The model under review builds one solid part; all positions refer to its coordinate system, in mm. Round coordinates to 2 decimals unless told otherwise and drop trailing zeros. Loops run counter-clockwise (first coordinate to the right, second up) from the corner with the lowest first, then second, coordinate; pieces in that order, holes last. Notation, with made-up numbers: (30.25, 46) -> (68.25, 46) arc R19 cw to (68.25, 69) -> close; hole circle Ø6 at (11, 82). An arc over 180 degrees is marked (long way). Write each question's results on one line, items separated by ' | '. Start each with the question number.
Item 1: We need section C-C (x = -43). Give the boundary of the cut face in (y, z).
Item 2: We need section D-D (z = 76). Give the boundary of the cut face in (x, y), and give its area (3 significant figures).
Item 3: We need section B-B (y = 0.65). Give the number of separate pieces and of enclosed holes in the cut face, and give its area (3 significant figures).
Item 4: For L1, parallel to X at y = 0.6, z = 92.5; L2, parallel to Z at x = 75.5, y = 2.1; L3, parallel to Z at x = -77.5, y = 0.3, list the stretches that pass through material, from the lowest coordinate up. Write a range as from..to.
Item 5: We need section A-A (z = -55). Give the boundary of the cut face in (x, y), and give its area (3 significant figures).
Item 6: Clearance check with flat-ended pins moving along their axes: pin 1 Ø1 at (y, z) = (1, 59.5) entering from +X; pin 2 Ø0.8 at (x, y) = (5, 1.5) entering from -Z; pin 3 Ø0.8 at (y, z) = (1, -76.5) entering from +X. State where each tip first meets the part, or that it passes through.
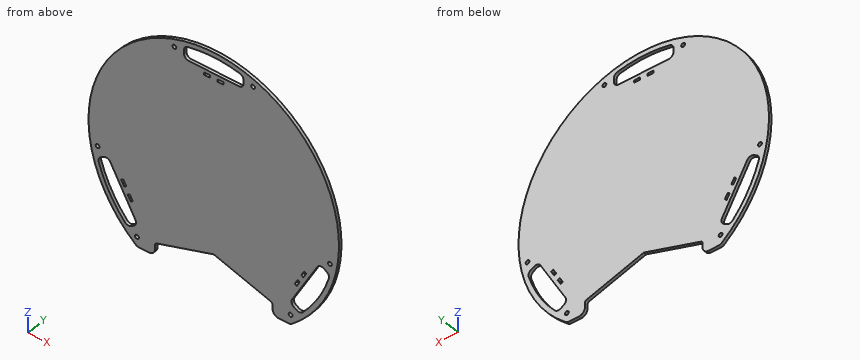
Autodesk Inventor part; units mm, degrees
ref_plane "YZ Plane" through (0, 0, 0) normal (1, 0, 0) x (0, 1, 0)
ref_plane "XZ Plane" through (0, 0, 0) normal (0, 1, 0) x (-1, 0, 0)
ref_plane "XY Plane" through (0, 0, 0) normal (0, 0, 1) x (1, 0, 0)
sketch "Sketch1" plane through (0, 0, 0) normal (0, 1, 0) x (-1, 0, 0)
  line L0 (-62.9285, -83) -> (-54.3117, -83)
  line L1 (62.9285, -83) -> (54.3117, -83)
  arc A0 (65.4207, -82.1287) -> (-65.4207, -82.1287) centre (0, 0) ccw
  line L2 (-49.3117, -78) -> (-49.3117, -74.4821)
  line L3 (-47.8938, -72.5687) -> (0, -58)
  line L4 (49.3117, -78) -> (49.3117, -74.4821)
  line L5 (47.8938, -72.5687) -> (0, -58)
  arc A1 (49.3117, -78) -> (54.3117, -83) centre (54.3117, -78) ccw
  arc A2 (-54.3117, -83) -> (-49.3117, -78) centre (-54.3117, -78) ccw
  arc A3 (49.3117, -74.4821) -> (47.8938, -72.5687) centre (47.3117, -74.4821) ccw
  arc A4 (-47.8938, -72.5687) -> (-49.3117, -74.4821) centre (-47.3117, -74.4821) ccw
  arc A5 (62.9285, -83) -> (65.4207, -82.1287) centre (62.9285, -79) ccw
  arc A6 (-65.4207, -82.1287) -> (-62.9285, -83) centre (-62.9285, -79) ccw
  line L6 (-76.2102, -44) -> (-65.7102, -62.1865)
  line L7 (-67.1743, -67.6506) -> (-69.6351, -69.0713)
  line L8 (-94.6351, -25.7701) -> (-92.1743, -24.3494)
  line L9 (-86.7102, -25.8135) -> (-76.2102, -44)
  arc A7 (-96.4496, -30.438) -> (-74.5849, -68.3088) centre (0, 0) ccw
  arc A8 (-94.6351, -25.7701) -> (-96.4496, -30.438) centre (-92.6351, -29.2342) ccw
  arc A9 (-86.7102, -25.8135) -> (-92.1743, -24.3494) centre (-90.1743, -27.8135) ccw
  arc A10 (-67.1743, -67.6506) -> (-65.7102, -62.1865) centre (-69.1743, -64.1865) ccw
  arc A11 (-74.5849, -68.3088) -> (-69.6351, -69.0713) centre (-71.6351, -65.6072) ccw
  line L10 (76.2102, -44) -> (86.7102, -25.8135)
  line L11 (92.1743, -24.3494) -> (94.6351, -25.7701)
  line L12 (69.6351, -69.0713) -> (67.1743, -67.6506)
  line L13 (65.7102, -62.1865) -> (76.2102, -44)
  arc A12 (74.5849, -68.3088) -> (96.4496, -30.438) centre (0, 0) ccw
  arc A13 (69.6351, -69.0713) -> (74.5849, -68.3088) centre (71.6351, -65.6072) ccw
  arc A14 (65.7102, -62.1865) -> (67.1743, -67.6506) centre (69.1743, -64.1865) ccw
  arc A15 (92.1743, -24.3494) -> (86.7102, -25.8135) centre (90.1743, -27.8135) ccw
  arc A16 (96.4496, -30.438) -> (94.6351, -25.7701) centre (92.6351, -29.2342) ccw
  line L14 (0, 88) -> (-21, 88)
  line L15 (-25, 92) -> (-25, 94.8414)
  line L16 (25, 94.8414) -> (25, 92)
  line L17 (21, 88) -> (0, 88)
  arc A17 (21.8647, 98.7468) -> (-21.8647, 98.7468) centre (0, 0) ccw
  arc A18 (25, 94.8414) -> (21.8647, 98.7468) centre (21, 94.8414) ccw
  arc A19 (21, 88) -> (25, 92) centre (21, 92) ccw
  arc A20 (-25, 92) -> (-21, 88) centre (-21, 92) ccw
  arc A21 (-21.8647, 98.7468) -> (-25, 94.8414) centre (-21, 94.8414) ccw
  circle A22 centre (-33, 93.4207) radius 1.6
  circle A23 centre (33, 93.4207) radius 1.6
  line L18 (-75.1122, -39.9019) -> (-77.6122, -35.5718)
  line L19 (-77.6122, -35.5718) -> (-75.8801, -34.5718)
  line L20 (-75.8801, -34.5718) -> (-73.3801, -38.9019)
  line L21 (-73.3801, -38.9019) -> (-75.1122, -39.9019)
  line L22 (-72.1122, -45.0981) -> (-69.6122, -49.4282)
  line L23 (-69.6122, -49.4282) -> (-67.8801, -48.4282)
  line L24 (-67.8801, -48.4282) -> (-70.3801, -44.0981)
  line L25 (-70.3801, -44.0981) -> (-72.1122, -45.0981)
  line L26 (72.1122, -45.0981) -> (69.6122, -49.4282)
  line L27 (69.6122, -49.4282) -> (67.8801, -48.4282)
  line L28 (67.8801, -48.4282) -> (70.3801, -44.0981)
  line L29 (70.3801, -44.0981) -> (72.1122, -45.0981)
  line L30 (73.3801, -38.9019) -> (75.1122, -39.9019)
  line L31 (75.8801, -34.5718) -> (73.3801, -38.9019)
  line L32 (77.6122, -35.5718) -> (75.8801, -34.5718)
  line L33 (75.1122, -39.9019) -> (77.6122, -35.5718)
  line L34 (3, 85) -> (8, 85)
  line L35 (8, 85) -> (8, 83)
  line L36 (8, 83) -> (3, 83)
  line L37 (3, 83) -> (3, 85)
  line L38 (-3, 83) -> (-3, 85)
  line L39 (-8, 83) -> (-3, 83)
  line L40 (-8, 85) -> (-8, 83)
  line L41 (-3, 85) -> (-8, 85)
  circle A24 centre (-64.4047, -75.2892) radius 1.6
  circle A25 centre (-97.4047, -18.1315) radius 1.6
  circle A26 centre (97.4047, -18.1315) radius 1.6
  circle A27 centre (64.4047, -75.2892) radius 1.6
  point P0 (64.3117, -83)
  point P1 (-64.3117, -83)
  point P2 (-49.3117, -83)
  point P3 (49.3117, -83)
  point P4 (-49.3117, -73)
  point P5 (49.3117, -73)
  point P6 (-63.7102, -65.6506)
  point P7 (-72.3705, -70.6506)
  point P8 (-97.3705, -27.3494)
  point P9 (88.7102, -22.3494)
  point P10 (97.3705, -27.3494)
  point P11 (-25, 88)
  point P12 (-25, 98)
  dimension "d65" = 360
  dimension "d68" = 3.2
  dimension "d70" = 3.2
  dimension "d79" = 360
  dimension "d83" = 360
extrude "Extrusion1" add sketch "Sketch1" along normal blind 2.5
properties part number "Bottom Plate"
Here are the results:
1) outline: (0, -71.08) -> (2.5, -71.08) -> (2.5, 95.79) -> (0, 95.79) -> close
2) outline: (-72.45, 0) -> (72.45, 0) -> (72.45, 2.5) -> (-72.45, 2.5) -> close | area: 362 mm2
3) separate pieces: 1 | enclosed holes: 15 | area: 29,100 mm2
4) L1: x = -49.69..-34.31, -31.69..-25, 25..31.69, 34.31..49.69 | L2: z = -72.97..-67.3, -45.23..-39.23, -35.23..72.97 | L3: z = -70.84..-64.98, -41.77..-35.77, -35.51..70.84
5) outline: (-89.44, 0) -> (-84.88, 0) -> (-84.88, 2.5) -> (-89.44, 2.5) -> close; (-69.86, 0) -> (69.86, 0) -> (69.86, 2.5) -> (-69.86, 2.5) -> close; (84.88, 0) -> (89.44, 0) -> (89.44, 2.5) -> (84.88, 2.5) -> close | area: 372 mm2
6) pin 1: stops at x = 86.86 | pin 2: stops at z = -59.64 | pin 3: stops at x = 72.34
